Can you work these out from the drawing? Everything is in mm from the part's minimum corner. Give positions to 0.01 mm unless a question says otherwise; leave off trailing zeros. Write each loop counter-clockwise with the first axis right and the second up, starting at its lowest first coordinate (ties: lowest second). Pieces come first, ordered by that corner, then holes. Notation, with made-up numbers: (28, -24) -> (81, -24) arc R17 cw to (81, -7) -> close; hole circle Ø8 at (83.5, 82.25). An arc over 180 degrees is marked (long way). Use one line per item in the form item = value.
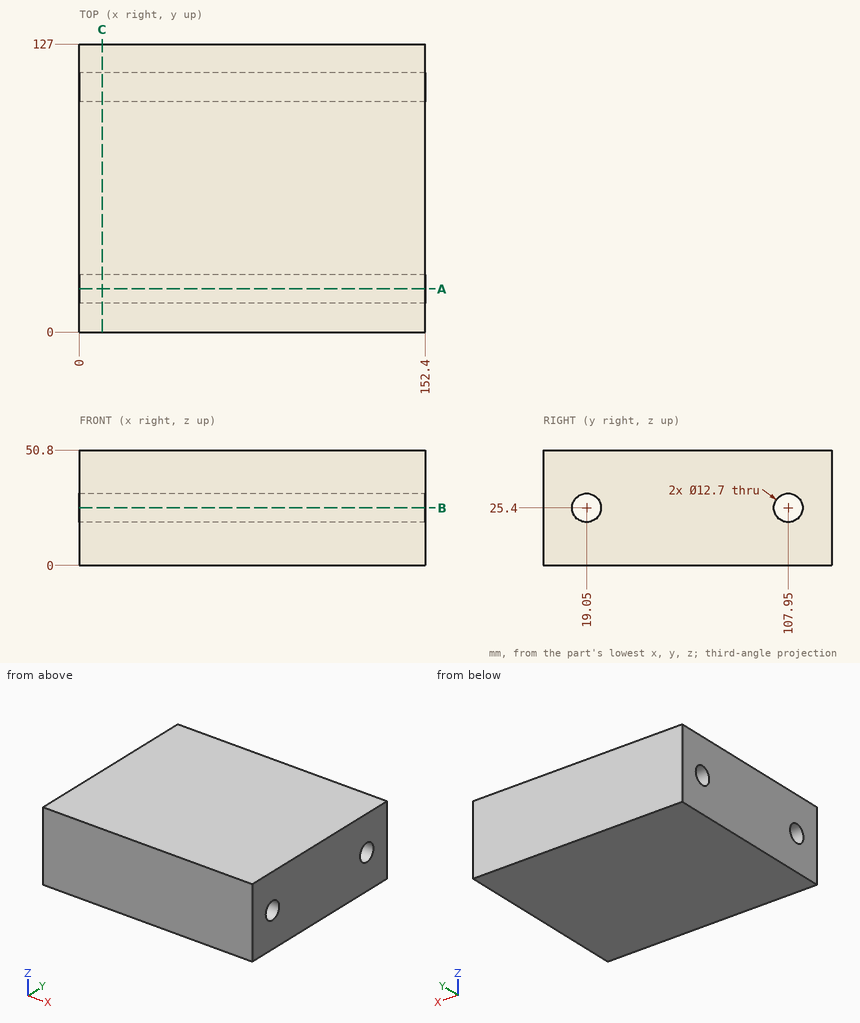
Q1. I want a section at A-A, the plane y = 19.05. Write out the boundary of the cut face in (x, z), and give its area (3 significant figures).
Result set:
outline = (0, 0) -> (152.4, 0) -> (152.4, 19.05) -> (0, 19.05) -> close; (0, 31.75) -> (152.4, 31.75) -> (152.4, 50.8) -> (0, 50.8) -> close
area = 5,810 mm2
Q2. If I drill on line 1 along Y through (x, z) = (103, 25.4); line 2 along Z through (x, y) = (47, 19); line 3 along Y through (x, z) = (78, 22.5), over which ranges is the centre line in solid material (lowest first)? Write a range as from..to.
Result set:
line_1 = 0..12.7, 25.4..101.6, 114.3..127
line_2 = 0..19.05, 31.75..50.8
line_3 = 0..13.4, 24.7..102.3, 113.6..127
Q3. Will this pin go through, and if not, where does the flat tip stop? pin 1 Ø10 at (y, z) = (107.95, 25.4) entering from +X.
Result set:
pin_1 = through
Q4. I want a section at B-B, the plane z = 25.4. Write out the boundary of the cut face in (x, y), and give its area (3 significant figures).
Result set:
outline = (0, 0) -> (152.4, 0) -> (152.4, 12.7) -> (0, 12.7) -> close; (0, 25.4) -> (152.4, 25.4) -> (152.4, 101.6) -> (0, 101.6) -> close; (0, 114.3) -> (152.4, 114.3) -> (152.4, 127) -> (0, 127) -> close
area = 15,500 mm2
Q5. I want a section at C-C, the plane x = 10. Write out the boundary of the cut face in (y, z).
Result set:
outline = (0, 0) -> (127, 0) -> (127, 50.8) -> (0, 50.8) -> close; hole circle Ø12.7 at (19.05, 25.4); hole circle Ø12.7 at (107.95, 25.4)
